```python
from build123d import *

# Parameters (mm, degrees)
F1_DEPTH  = 24
F2_W      = 48
F2_H      = 12.7
F2_H_2    = 19.05
F3_DEPTH  = 12.7
F4_R      = 9.525
F6_R      = 9.525
F8_DEPTH  = 47.498
F10_DEPTH = 25.4
F5_W      = 48
F5_H      = 19.05
F5_H_2    = 12.7
F11_DEPTH = 12.7
F12_R     = 9.525
F15_DEPTH = 25.4


# Not quite as in the source:
# - two fillets or chamfers of one size are made in one step
# - a feature names something its author has since deleted; it is built from what else it names


with BuildPart() as f1:
    # F0 (on Right) → F1 (new body, symmetric)
    with BuildSketch(Plane.YZ):
        with BuildLine():
            ThreePointArc((-34.925, 0), (0, 34.925), (34.925, 0))
            Line((34.925, 0), (98.425, 0))
            Line((98.425, 0), (98.425, 12.7))
            Line((98.425, 12.7), (87.425, 12.7))
            Line((87.425, 12.7), (45.900442536, 12.7))
            ThreePointArc((45.900442536, 12.7), (0, 47.625), (-45.900442536, 12.7))
            Line((-45.900442536, 12.7), (-98.425, 12.7))
            Line((-98.425, 12.7), (-98.425, 0))
            Line((-98.425, 0), (-34.925, 0))
        make_face()
    extrude(amount=F1_DEPTH, both=True)

    # F2 (on face) → F3 (join)
    with BuildSketch(Plane.XZ.offset(98.425)):
        with Locations((0, 6.35)):
            Rectangle(F2_W, F2_H)
        with Locations((0, -9.525)):
            Rectangle(F2_W, F2_H_2)
    extrude(amount=F3_DEPTH)

    # F4
    f4_edges = [f1.edges().sort_by_distance(p)[0] for p in [
        (0, -111.125, 12.7),
    ]]
    fillet(f4_edges, radius=F4_R)

    # F6
    f6_edges = [f1.edges().sort_by_distance(p)[0] for p in [
        (0, -45.900443, 12.7),
        (0, 45.900443, 12.7),
    ]]
    fillet(f6_edges, radius=F6_R)

    # F7 (on face) → F8 (cut)
    with BuildSketch(Plane(origin=(0, 0, 0), x_dir=(1, 0, 0), z_dir=(0, 0, -1))):
        with BuildLine():
            ThreePointArc((9.525, 76.2), (-6.7351920908, 82.9351920908), (0, 66.675))
            ThreePointArc((0, 66.675), (6.7351920908, 69.4648079092), (9.525, 76.2))
        make_face()
    extrude(amount=-F8_DEPTH, mode=Mode.SUBTRACT)

    # F9 (on face) → F10 (cut)
    with BuildSketch(Plane(origin=(0, 0, 0), x_dir=(1, 0, 0), z_dir=(0, 0, -1))):
        with BuildLine():
            ThreePointArc((9.525, -6.35), (6.7351920908, 0.3851920908), (0, 3.175))
            ThreePointArc((0, 3.175), (-6.7351920908, -13.0851920908), (9.525, -6.35))
        make_face()
    extrude(amount=-F10_DEPTH, mode=Mode.SUBTRACT)

    # F5 (on face) → F11 (join)
    with BuildSketch(Plane(origin=(0, 98.425, 0), x_dir=(-1, 0, 0), z_dir=(0, 1, 0))):
        with Locations((0, -9.525)):
            Rectangle(F5_W, F5_H)
        with Locations((0, 6.35)):
            Rectangle(F5_W, F5_H_2)
    extrude(amount=F11_DEPTH)

    # F12
    f12_edges = [f1.edges().sort_by_distance(p)[0] for p in [
        (0, 111.125, 12.7),
    ]]
    fillet(f12_edges, radius=F12_R)

    # F14 (on face) → F15 (cut)
    with BuildSketch(Plane(origin=(0, 0, 0), x_dir=(1, 0, 0), z_dir=(0, 0, -1))):
        with BuildLine():
            ThreePointArc((9.525, -76.2), (6.7351920908, -69.4648079092), (0, -66.675))
            ThreePointArc((0, -66.675), (-6.7351920908, -82.9351920908), (9.525, -76.2))
        make_face()
    extrude(amount=-F15_DEPTH, mode=Mode.SUBTRACT)


solid = f1.part
```
Source: CAD feature listing. Evaluate the final solid. Frame: model axes, mm. A direction names the side the tool comes from. Round coordinates to 2 decimals unless told otherwise and drop trailing zeros. Loops run counter-clockwise (first coordinate to the right, second up) from the corner with the lowest first, then second, coordinate; pieces in that order, holes last.
1. Section query A-A on z = 6.5. Output: boundary loops of the cut face in (x, y) (3 decimals).
2. Section query B-B on y = 76.2. Output: boundary loops of the cut face in (x, z) (3 decimals), and give its area (3 significant figures).
3. Section query D-D on x = -11.5. Output: boundary loops of the cut face in (y, z) (3 decimals).
4. Access query for faces 4 (the flat face through (10, -77, 12.7)), 5 (the flat face through (0, 66, 0)), 6 (the flat face through (-10, 77, 12.7)), 7 (the cylindrical face through (3.65, 67.4, 6.26)). Directions: +Z, -Z, +X, -X, +Y, -Y. A direction counts if a zero-diameter tool reaches every point of the face in a straight line with its end or side. Return the directions, or none.
5. Section query C-C on z = -6. Output: boundary loops of the cut face in (x, y) (3 decimals), and give its area (3 significant figures).
6. Contact query for flat-ended pins moving along their axis: pin 1 (24 mm diameter, centred on x = 7.5, y = 73.5, fed in from +Z); pin 2 (8 mm diameter, centred on x = 13.5, z = 32, fed in from -Y); pin 3 (1.5 mm diameter, centred on x = 6.5, y = -23, fed in from +Z); pin 4 (11.5 mm diameter, centred on x = 0, y = -76.2, fed in from -Z). Output: stop coordinate, or through.
7. Mould query, pull axis Y, two halves, no side actions, for faces 1 (the cylindrical face through (-3.65, -67.4, 6.26)), 2 (the cylindrical face through (0.34, 47.32, 14.33)), 3 (the cylindrical face through (0.34, 0.78, 47.62)). Classes: released by +Y, released by -Y, zero draft, split by the parting line, or undercut.
8. Ray query, L1, parallel to X at y = -76.2, z = 3.75 (3 decimals); L2, parallel to Y at x = 11, z = 1.5 (3 decimals); L3, parallel to Y at x = -1, z = 3 (3 decimals). Return the intervals inside material, ascending.
Answers below:
1. outline: (-24, -110.526) - (24, -110.526) - (24, -34.315) - (-24, -34.315) - close; (-24, 34.315) - (24, 34.315) - (24, 110.526) - (-24, 110.526) - close; hole circle Ø19.05 at (0, -76.2); hole circle Ø19.05 at (0, 76.2)
2. outline: (-24, 0) - (-9.525, 0) - (-9.525, 12.7) - (-24, 12.7) - close; (9.525, 0) - (24, 0) - (24, 12.7) - (9.525, 12.7) - close
2. area: 368 mm2
3. outline: (-111.125, -19.05) - (-98.425, -19.05) - (-98.425, 0) - (-34.925, 0) arc R34.925 cw to (34.925, 0) - (98.425, 0) - (98.425, -19.05) - (111.125, -19.05) - (111.125, 3.175) arc R9.525 ccw to (101.6, 12.7) - (52.651, 12.7) arc R9.525 cw to (43.876, 18.521) arc R47.625 ccw to (-43.876, 18.521) arc R9.525 cw to (-52.651, 12.7) - (-101.6, 12.7) arc R9.525 ccw to (-111.125, 3.175) - close
4. face 4: +Z, +X, -X, -Y
4. face 5: -Z, +X, -X
4. face 6: +Z, +X, -X, +Y
4. face 7: +Z, -Z
5. outline: (-24, -111.125) - (24, -111.125) - (24, -98.425) - (-24, -98.425) - close; (-24, 98.425) - (24, 98.425) - (24, 111.125) - (-24, 111.125) - close
5. area: 1,220 mm2
6. pin 1: stops at z = 12.7
6. pin 2: stops at y = -38.52
6. pin 3: stops at z = 42.11
6. pin 4: passes through
7. face 1: undercut
7. face 2: released by +Y
7. face 3: split by the parting line
8. L1: x = -24 to -9.525, 9.525 to 24
8. L2: y = -111.125 to -34.893, 34.893 to 111.125
8. L3: y = -111.125 to -85.672, -66.728 to -34.796, 34.796 to 66.728, 85.672 to 111.125
